Build history of the part. All positions in model axes, mm. Face numbers are marked on the shaded views. A direction names the side the tool comes from. Round coordinates to 2 decimals unless told otherwise and drop trailing zeros. Loops run counter-clockwise (first coordinate to the right, second up) from the corner with the lowest first, then second, coordinate; pieces in that order, holes last. Notation, with made-up numbers: (86.25, -2.75) - (102.25, -2.75) arc R21 cw to (102.25, 1.25) - close; hole circle Ø3 at (49, -6). An arc over 180 degrees is marked (long way). Answer as CSV lines item,"result". Start each with the question number.
Autodesk Fusion 360 part; units mm, degrees
sketch "Sketch1" plane through (0, 0, 0) normal (1, 0, 0) x (0, 1, 0)
  line L0 (0, 0) -> (-70, 0)
  line L1 (-70, 0) -> (-70, 50)
  line L2 (-70, 50) -> (0, 50)
  line L3 (0, 50) -> (0, 0)
  dimension "d1" = 70
  dimension "d2" = 50
extrude "Extrude1" add sketch "Sketch1" along normal blind 50
fillet "Fillet1" radius 5 4 edges at (25, 0, 50) (25, 0, 0) (25, -70, 0) (25, -70, 50)
shell "Shell1" thickness 2 removed faces 1 at (50, -45, 16.6667)
extrude "Extrude3" add 1 faces at (0, -45, 16.6667) along direction (-1, 0, 0) blind 2
extrude "Extrude4" cut 1 faces at (2, -25, 17.3333) along direction (-1, 0, 0) blind 3
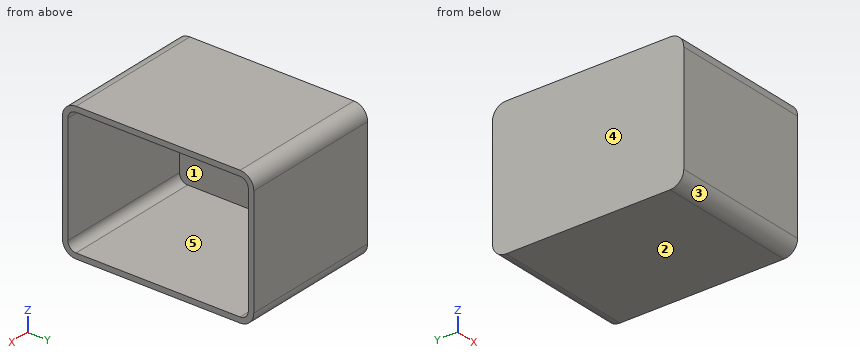
Q1. Wall check: probe 1 along Y at (x, z) = (8, 12); probe 2 along Z at (x, y) = (27, -64); probe 3 along X at (y, z) = (-49.5, 36). Give the ranges that are in metal, low to high. Write a range as [from, to].
Q2. Two-plate mould, pull along Y, no slides. Class the marked faces 3, 4 and 5: released by +Y, released by -Y, zero draft, split by the parting line, or undercut.
Q3. Band-saw the part on C-C, the plane y = -49.5. List the corners of the cut face in (x, z).
Q4. Band-saw the part on B-B, the plane x = 47. List the corners of the cut face in (y, z), then the cut area to 3 significant figures.
Q5. Pin check, flat tips, straight feed: pin 1 Ø20 at (x, z) = (30.5, 22.5) entering from +Y; pin 2 Ø23 at (y, z) = (-20, 31.5) entering from +X. Stop position of each tip, or through.
Q6. Band-saw the part on A-A, the plane z = 17. List the corners of the cut face in (x, y), then the cut area to 3 significant figures.
Q7. Tool access for the marked faces 1 and 2: list every direction of +Z, -Z, +X, -X, +Y, -Y with a clear straight run to the whole face (end or side of a thin tool).
Reported:
1,probe 1,"y = [-70, -68], [-2, 0]"
1,probe 2,"z = [0, 2], [48, 50]"
1,probe 3,"x = [-2, -1]"
2,face 3,"released by -Y"
2,face 4,"zero draft"
2,face 5,"undercut"
3,outline,"(-2, 0) - (50, 0) - (50, 2) - (-1, 2) - (-1, 48) - (50, 48) - (50, 50) - (-2, 50) - close"
4,outline,"(-70, 5) arc R5 ccw to (-65, 0) - (-5, 0) arc R5 ccw to (0, 5) - (0, 45) arc R5 ccw to (-5, 50) - (-65, 50) arc R5 ccw to (-70, 45) - close; hole (-68, 5) arc R3 ccw to (-65, 2) - (-5, 2) arc R3 ccw to (-2, 5) - (-2, 45) arc R3 ccw to (-5, 48) - (-65, 48) arc R3 ccw to (-68, 45) - close"
4,area,"450 mm2"
5,pin 1,"stops at y = 0"
5,pin 2,"stops at x = -1"
6,outline,"(-2, -70) - (50, -70) - (50, -68) - (-1, -68) - (-1, -2) - (50, -2) - (50, 0) - (-2, 0) - close"
6,area,"274 mm2"
7,face 1,"+X"
7,face 2,"-Z, +X, -X, +Y, -Y"
